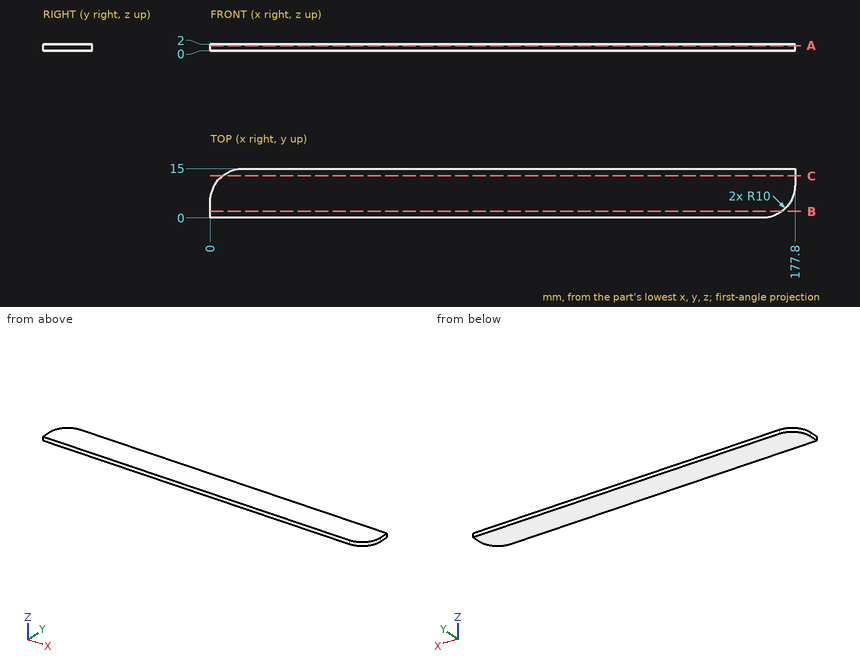
Study the drawing (mm; zero at the part's minimum x, y, z) and answer. Coordinates: 2 decimals unless noted, no trailing zeros. Write each loop counter-clockwise with the first axis right and the second up, starting at its lowest first coordinate (ties: lowest second). Pieces come first, ordered by that corner, then holes.
Q1. Find the intervals of material crossed by line 1 along X through (y, z) = (11.25, 0.7); line 2 along X through (y, z) = (9.75, 0.5); line 3 along Y through (x, z) = (170, 0.35) (3 decimals), in increasing order.
Returned:
line 1: x = 2.19 to 177.8
line 2: x = 1.2 to 177.8
line 3: y = 0.245 to 15
Q2. Section A-A, the plane z = 1.5 is taken. Write down the section's boundary in (x, y), then the cut area to 3 significant figures.
Returned:
outline: (0, 0) - (167.8, 0) arc R10 ccw to (177.8, 10) - (177.8, 15) - (10, 15) arc R10 ccw to (0, 5) - close
area: 2,620 mm2
Q3. Section B-B, the plane y = 2 is taken. Write down the section's boundary in (x, z).
Returned:
outline: (0, 0) - (173.8, 0) - (173.8, 2) - (0, 2) - close
Q4. Given P1, Ø1, axis at y = 4, z = 1, coming from the +X side, flat-ended and moving along its own axis, determine where the tip first touches the part or whether it passes through.
Returned:
P1: stops at x = 176.15
Q5. Section C-C, the plane y = 12.75 is taken. Write down the section's boundary in (x, z).
Returned:
outline: (3.68, 0) - (177.8, 0) - (177.8, 2) - (3.68, 2) - close
